```python
from build123d import *

# Parameters (mm, degrees)
SKETCH1_R           = 58
SKETCH1_R_2         = 6.625
BOSS_EXTRUDE1_DEPTH = 3
SKETCH2_R           = 7.6
CUT_EXTRUDE1_DEPTH  = 2


with BuildPart() as part:
    # Sketch1 → Boss-Extrude1 (new body)
    with BuildSketch(Plane(origin=(0, 0, 0), x_dir=(1, 0, 0), z_dir=(0, 1, 0))):
        Circle(SKETCH1_R)
        with Locations((0, 48.699495206)):
            Circle(SKETCH1_R_2, mode=Mode.SUBTRACT)
        with Locations((42.175, -24.349747603)):
            Circle(SKETCH1_R_2, mode=Mode.SUBTRACT)
        with Locations((-42.175, -24.349747603)):
            Circle(SKETCH1_R_2, mode=Mode.SUBTRACT)
    extrude(amount=BOSS_EXTRUDE1_DEPTH)

    # Sketch2 → Cut-Extrude1 (cut)
    with BuildSketch(Plane.XZ):
        with Locations((42.175, 24.349747603)):
            Circle(SKETCH2_R)
        with Locations((-42.175, 24.349747603)):
            Circle(SKETCH2_R)
        with Locations((0, -48.699495206)):
            Circle(SKETCH2_R)
    extrude(amount=-CUT_EXTRUDE1_DEPTH, mode=Mode.SUBTRACT)


solid = part.part
```
Part model, mm, in its own coordinate system. A direction names the side the tool comes from. Give positions to 0.01 mm unless a question says otherwise; leave off trailing zeros. Write each loop counter-clockwise with the first axis right and the second up, starting at its lowest first coordinate (ties: lowest second). Pieces come first, ordered by that corner, then holes. Notation, with made-up numbers: (84.5, -3.5) -> (120.5, -3.5) arc R10 cw to (120.5, 10.5) -> close; hole circle Ø3 at (-37.75, -2.75). An arc over 180 degrees is marked (long way). Put each result on its own line as item: value. Start each with the question number.
Item 1: Which spindle directions (+Z, -Z, +X, -X, +Y, -Y) get a long thin tool onto all of the face, cutting with end or side? Do faces 1 (the face through (-0.86, 2.49, -55.27)), 2 (the face through (-2, 2, -42)). Say none if no direction does.
Item 2: Pull direction Z, two halves, no side cores. Call faces 3 (the face through (26.76, 1.48, 51.46)), 4 (the face through (-35.856, 2.493, 22.36)), 5 (the face through (-1, 0, -1)): pulls with the +Z half, pulls with the -Z half, needs draft (parallel to the pull), parting line crosses it, or undercut.
Item 3: Cut at B-B (z = -46.5). List the corners of the cut face in (x, y), then the cut area to 3 significant figures.
Item 4: Cut at C-C (y = 1.55). List the corners of the cut face in (x, z) (1 decimal).
Item 5: Pin check, flat tips, straight feed: pin 1 Ø6 at (x, z) = (-33.5, -44.5) entering from -Y; pin 2 Ø15 at (x, z) = (-42.18, 24.35) entering from -Y. Stop position of each tip, or through.
Item 6: Cut at D-D (x = -31). List the corners of the cut face in (y, z), then the cut area to 3 significant figures.
Item 7: Wall check: L1, parallel to X at y = 0.4, z = 25.5; L2, parallel to X at y = 1.8, z = 30.5; L3, parallel to Z at x = 0, y = 0.3. Give the ranges that are in metal, low to high. Write a range as [from, to].
Item 8: Cut at A-A (x = 0). List the corners of the cut face in (y, z).
Answer list:
1. face 1: +Y, -Y
1. face 2: -Y
2. face 3: parting line crosses it
2. face 4: undercut
2. face 5: needs draft
3. outline: (-34.67, 0) -> (-7.27, 0) -> (-7.27, 2) -> (-6.25, 2) -> (-6.25, 3) -> (-34.67, 3) -> close; (6.25, 2) -> (7.27, 2) -> (7.27, 0) -> (34.67, 0) -> (34.67, 3) -> (6.25, 3) -> close
3. area: 166 mm2
4. outline: circle Ø116 at (0, 0); hole circle Ø15.2 at (-42.2, 24.3); hole circle Ø15.2 at (0, -48.7); hole circle Ø15.2 at (42.2, 24.3)
5. pin 1: stops at y = 0
5. pin 2: stops at y = 2
6. outline: (0, -49.02) -> (3, -49.02) -> (3, 49.02) -> (0, 49.02) -> close
6. area: 294 mm2
7. L1: x = [-52.09, -49.69], [-34.66, 34.66], [49.69, 52.09]
7. L2: x = [-49.33, -46.64], [-37.71, 37.71], [46.64, 49.33]
7. L3: z = [-58, -56.3], [-41.1, 58]
8. outline: (0, -58) -> (3, -58) -> (3, -55.32) -> (2, -55.32) -> (2, -56.3) -> (0, -56.3) -> close; (0, -41.1) -> (2, -41.1) -> (2, -42.07) -> (3, -42.07) -> (3, 58) -> (0, 58) -> close
